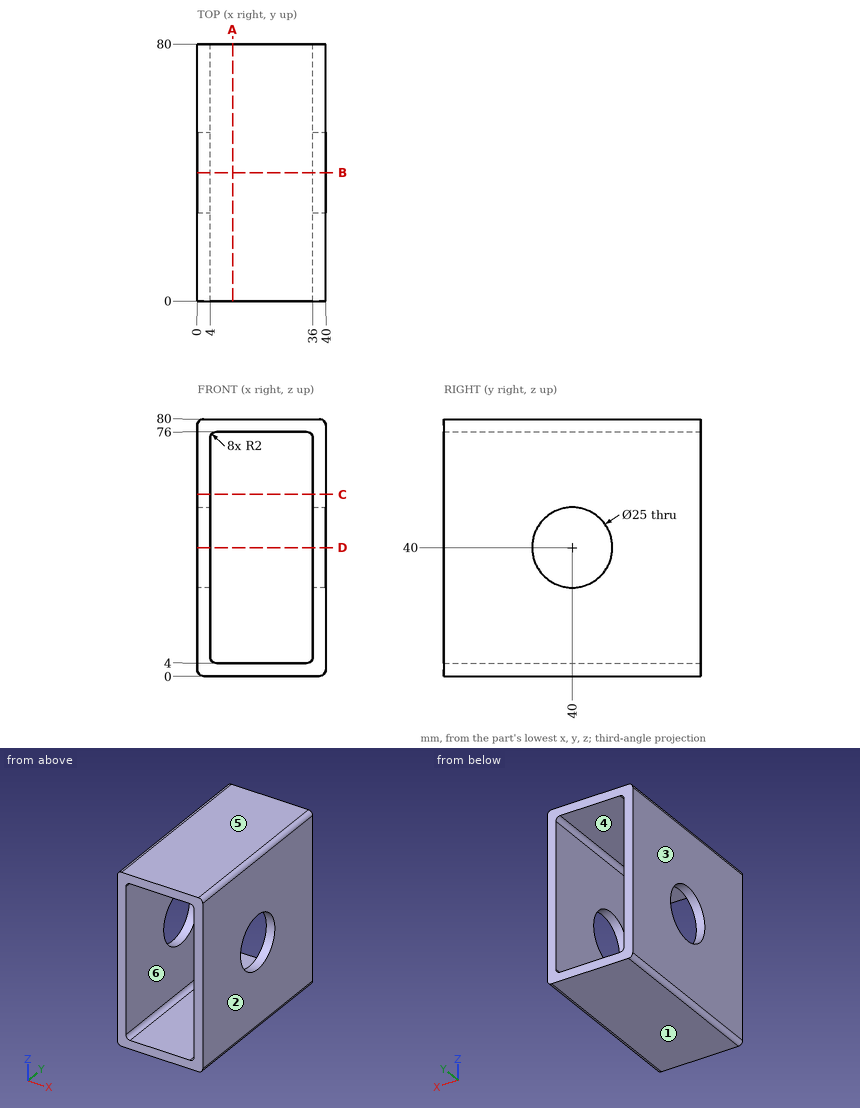
Could you check a few things on this drawing? It's one solid part, dimensions in mm from its lowest x, y, z. A direction names the side the tool comes from. Give positions to 0.01 mm unless a question says otherwise; leave off trailing zeros. Write each loop counter-clockwise with the first axis right and the second up, starting at its lowest first coordinate (ties: lowest second). Pieces come first, ordered by that corner, then holes. Notation, with made-up numbers: (59, 68) -> (79, 68) arc R34 cw to (79, 103) -> close; hole circle Ø2 at (77, 64.25). An arc over 180 degrees is marked (long way). Answer as CSV lines item,"result". Start each with the question number.
(1) If we section it at C-C, the plane z = 56.5: Write out the boundary of the cut face in (x, y), and give its area (3 significant figures).
(2) If we section it at B-B, the plane y = 40: Write out the boundary of the cut face in (x, z), and give its area (3 significant figures).
(3) Please list where these lines run through material, in increasing order: line 1 (Z direction, x = 26.5, y = 62); line 2 (X direction, y = 35, z = 23.5); line 3 (Y direction, x = 2.65, z = 40).
(4) Which directions (+Z, -Z, +X, -X, +Y, -Y) give clear straight access to the entire face, cutting with the end or side of a thin tool? Please do the marked faces 5 and 6.
(5) If we mould it in two halves opening along X, with no side actions, what happens to the marked faces 1, 2, 3 and 4? For each: +X half, -X half, draft (parallel to the pull), parting line (faces both ways), or undercut.
(6) If we section it at A-A, the plane x = 11: Write out the boundary of the cut face in (y, z).
(7) If we section it at D-D, the plane z = 40: Write out the boundary of the cut face in (x, y), and give its area (3 significant figures).
Answer list:
1,outline,"(0, 0) -> (4, 0) -> (4, 80) -> (0, 80) -> close; (36, 0) -> (40, 0) -> (40, 80) -> (36, 80) -> close"
1,area,"640 mm^2"
2,outline,"(0, 2) arc R2 ccw to (2, 0) -> (38, 0) arc R2 ccw to (40, 2) -> (40, 27.5) -> (36, 27.5) -> (36, 6) arc R2 cw to (34, 4) -> (6, 4) arc R2 cw to (4, 6) -> (4, 27.5) -> (0, 27.5) -> close; (0, 52.5) -> (4, 52.5) -> (4, 74) arc R2 cw to (6, 76) -> (34, 76) arc R2 cw to (36, 74) -> (36, 52.5) -> (40, 52.5) -> (40, 78) arc R2 ccw to (38, 80) -> (2, 80) arc R2 ccw to (0, 78) -> close"
2,area,"696 mm^2"
3,line 1,"0 to 4, 76 to 80"
3,line 2,"0 to 4, 36 to 40"
3,line 3,"0 to 27.5, 52.5 to 80"
4,face 5,"+Z, +X, -X, +Y, -Y"
4,face 6,"+Y, -Y"
5,face 1,"draft"
5,face 2,"+X half"
5,face 3,"-X half"
5,face 4,"undercut"
6,outline,"(0, 0) -> (80, 0) -> (80, 4) -> (0, 4) -> close; (0, 76) -> (80, 76) -> (80, 80) -> (0, 80) -> close"
7,outline,"(0, 0) -> (4, 0) -> (4, 27.5) -> (0, 27.5) -> close; (0, 52.5) -> (4, 52.5) -> (4, 80) -> (0, 80) -> close; (36, 0) -> (40, 0) -> (40, 27.5) -> (36, 27.5) -> close; (36, 52.5) -> (40, 52.5) -> (40, 80) -> (36, 80) -> close"
7,area,"440 mm^2"
